For this review, take the finished solid that the model builds, in its own axes (mm). Face numbers are marked on the shaded views. A direction names the side the tool comes from. Coordinates: 2 decimals unless noted, no trailing zeros. Loops run counter-clockwise (first coordinate to the right, second up) from the corner with the lowest first, then second, coordinate; pieces in that order, holes last. Notation, with made-up numbers: (-35, -30) -> (15, -30) arc R24 cw to (15, -17) -> close; hole circle Ø5 at (26.25, 11.5). An arc over 180 degrees is marked (long way). Use a Markdown table: item, result.
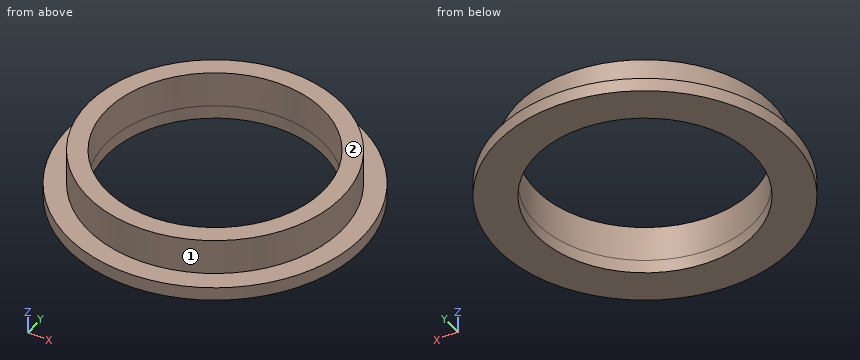
from build123d import *

# Parameters (mm, degrees)
F0_R     = 9.5
F0_R_2   = 8.125
F1_DEPTH = 2.65
F0_R_3   = 11
F2_DEPTH = 1


with BuildPart() as f1:
    # F0 (on Top) → F1 (new body)
    with BuildSketch(Plane.XY):
        Circle(F0_R)
        Circle(F0_R_2, mode=Mode.SUBTRACT)
    extrude(amount=F1_DEPTH)

    # F0 (on Top) → F2 (join)
    with BuildSketch(Plane.XY):
        Circle(F0_R_3)
        Circle(F0_R, mode=Mode.SUBTRACT)
        Circle(F0_R)
        Circle(F0_R_2, mode=Mode.SUBTRACT)
    extrude(amount=-F2_DEPTH)


solid = f1.part
(1) Take a section at D-D on x = 9. Write out the cut boundary in (y, z), plus the area to 3 significant figures.
Found:
| item | result |
|---|---|
| outline | (-6.32, -1) -> (6.32, -1) -> (6.32, 0) -> (3.04, 0) -> (3.04, 2.65) -> (-3.04, 2.65) -> (-3.04, 0) -> (-6.32, 0) -> close |
| area | 28.8 mm^2 |
(2) Take a section at C-C on z = -0.55. Write out the cut boundary in (x, y) (3 decimals).
Found:
| item | result |
|---|---|
| outline | circle Ø22 at (0, 0); hole circle Ø16.25 at (0, 0) |
(3) For pin 1 Ø3 at (x, y) = (-1, -5) entering from +Z; pin 2 Ø6.5 at (x, y) = (5, -2) entering from +Z; pin 3 Ø2 at (y, z) = (8.5, 0) entering from +X, all flat-tipped, find the tip position at first contact; note any pin that passes through.
Found:
| item | result |
|---|---|
| pin 1 | passes through |
| pin 2 | stops at z = 2.65 |
| pin 3 | stops at x = 8.05 |
(4) For line 1 along X through (y, z) = (0.25, -0.35); line 2 along Y through (x, z) = (0, 1.6) (3 decimals); line 3 along Y through (x, z) = (0, -0.5) (3 decimals), list the stretches that pass through material, from the lowest coordinate up.
Found:
| item | result |
|---|---|
| line 1 | x = -11 to -8.12, 8.12 to 11 |
| line 2 | y = -9.5 to -8.125, 8.125 to 9.5 |
| line 3 | y = -11 to -8.125, 8.125 to 11 |
(5) For the marked faces 1 and 2, list the 3-axis set-ups (+Z, -Z, +X, -X, +Y, -Y) from which the entire face can be reached by the end or side of a thin tool; tool diameter is ignored.
Found:
| item | result |
|---|---|
| face 1 | +Z |
| face 2 | +Z, +X, -X, +Y, -Y |
(6) Take a section at A-A on y = 0. Write out the cut boundary in (x, z) (3 decimals), plus the area to 3 significant figures.
Found:
| item | result |
|---|---|
| outline | (-11, -1) -> (-8.125, -1) -> (-8.125, 2.65) -> (-9.5, 2.65) -> (-9.5, 0) -> (-11, 0) -> close; (8.125, -1) -> (11, -1) -> (11, 0) -> (9.5, 0) -> (9.5, 2.65) -> (8.125, 2.65) -> close |
| area | 13.0 mm^2 |
